Read the model definition and answer for the solid it produces. Units are mm, in the model's axes. Face numbers are marked on the shaded views. A direction names the side the tool comes from. Coordinates: 2 decimals unless noted, no trailing zeros. Loops run counter-clockwise (first coordinate to the right, second up) from the corner with the lowest first, then second, coordinate; pieces in that order, holes last. Notation, with made-up numbers: M 11.25,45.5 L 58.25,45.5 A17 ccw 58.25,69.5 Z; hole C -33.5,62.25 d1. An arc over 180 degrees is marked long. Put each result on its own line as item: value.
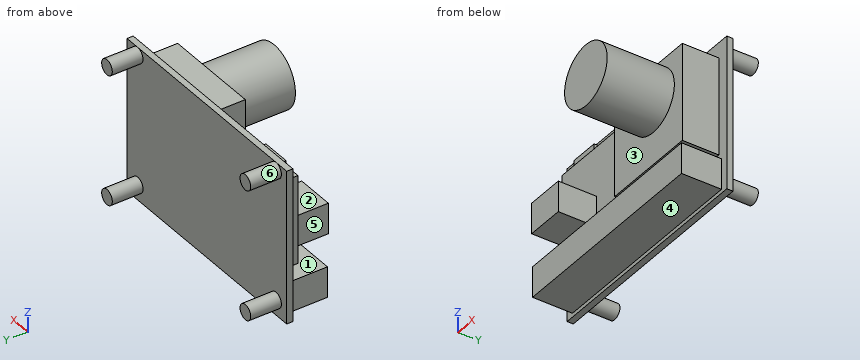
from build123d import *

# Parameters (mm, degrees)
P01_STANDOFF_START             = 28.6
SK_P01_STANDOFF_R              = 2
P01_STANDOFF_DEPTH             = 8
P02_STANDOFF_START             = 28.6
SK_P02_STANDOFF_R              = 2
P02_STANDOFF_DEPTH             = 8
P03_STANDOFF_START             = 28.6
SK_P03_STANDOFF_R              = 2
P03_STANDOFF_DEPTH             = 8
P04_STANDOFF_START             = 28.6
SK_P04_STANDOFF_R              = 2
P04_STANDOFF_DEPTH             = 8
P05_CARRIERBOARD_START         = 27
SK_P05_CARRIERBOARD_W          = 60
SK_P05_CARRIERBOARD_H          = 40
P05_CARRIERBOARD_DEPTH         = 1.6
P06_INA2602COMPUTE_START       = 24.3
SK_P06_INA2602COMPUTE_W        = 22.9
SK_P06_INA2602COMPUTE_H        = 23
P06_INA2602COMPUTE_DEPTH       = 2.7
P07_INA260TERMINALBLOCK_START  = 14.3
SK_P07_INA260TERMINALBLOCK_W   = 10
SK_P07_INA260TERMINALBLOCK_H   = 8
P07_INA260TERMINALBLOCK_DEPTH  = 10
P08_BUCKAD36V50F551V_START     = 17.5
SK_P08_BUCKAD36V50F551V_W      = 25.4
SK_P08_BUCKAD36V50F551V_H      = 25.4
P08_BUCKAD36V50F551V_DEPTH     = 9.5
P09_JSTXHHEADERSFACEDOWN_START = 16.6
SK_P09_JSTXHHEADERSFACEDOWN_W  = 56
SK_P09_JSTXHHEADERSFACEDOWN_H  = 8
P09_JSTXHHEADERSFACEDOWN_DEPTH = 10.4
P10_D2IDEALDIODE_START         = 24.6
SK_P10_D2IDEALDIODE_W          = 7.6
SK_P10_D2IDEALDIODE_H          = 12.7
P10_D2IDEALDIODE_DEPTH         = 2.4
SK_P11_C14700UF25V_R           = 8
P11_C14700UF25V_DEPTH          = 27


with BuildPart() as part:
    # SK_P01_Standoff → P01_Standoff (new body)
    with BuildSketch(Plane(origin=(0, 0, 0), x_dir=(1, 0, 0), z_dir=(0, 1, 0)).offset(P01_STANDOFF_START)):
        with Locations(Location((-26, -18, 0), (0, 0, 270))):
            Circle(SK_P01_STANDOFF_R)
    extrude(amount=P01_STANDOFF_DEPTH)



with BuildPart() as body_2:
    # SK_P02_Standoff → P02_Standoff (new body)
    with BuildSketch(Plane(origin=(0, 0, 0), x_dir=(1, 0, 0), z_dir=(0, 1, 0)).offset(P02_STANDOFF_START)):
        with Locations(Location((-26, 16, 0), (0, 0, 270))):
            Circle(SK_P02_STANDOFF_R)
    extrude(amount=P02_STANDOFF_DEPTH)


with BuildPart() as body_3:
    # SK_P03_Standoff → P03_Standoff (new body)
    with BuildSketch(Plane(origin=(0, 0, 0), x_dir=(1, 0, 0), z_dir=(0, 1, 0)).offset(P03_STANDOFF_START)):
        with Locations(Location((26, -18, 0), (0, 0, 270))):
            Circle(SK_P03_STANDOFF_R)
    extrude(amount=P03_STANDOFF_DEPTH)


with BuildPart() as body_4:
    # SK_P04_Standoff → P04_Standoff (new body)
    with BuildSketch(Plane(origin=(0, 0, 0), x_dir=(1, 0, 0), z_dir=(0, 1, 0)).offset(P04_STANDOFF_START)):
        with Locations(Location((26, 16, 0), (0, 0, 270))):
            Circle(SK_P04_STANDOFF_R)
    extrude(amount=P04_STANDOFF_DEPTH)


with BuildPart() as part_1:
    add(part.part)

    add(body_2.part)  # P05_Carrierboard merges body 2

    add(body_3.part)  # P05_Carrierboard merges body 3

    add(body_4.part)  # P05_Carrierboard merges body 4
    # SK_P05_Carrierboard → P05_Carrierboard (add)
    with BuildSketch(Plane(origin=(0, 0, 0), x_dir=(1, 0, 0), z_dir=(0, 1, 0)).offset(P05_CARRIERBOARD_START)):
        Rectangle(SK_P05_CARRIERBOARD_W, SK_P05_CARRIERBOARD_H)
    extrude(amount=P05_CARRIERBOARD_DEPTH)

    # SK_P06_INA2602compute → P06_INA2602compute (add)
    with BuildSketch(Plane(origin=(0, 0, 0), x_dir=(1, 0, 0), z_dir=(0, 1, 0)).offset(P06_INA2602COMPUTE_START)):
        with Locations((-16.55, -4.5)):
            Rectangle(SK_P06_INA2602COMPUTE_W, SK_P06_INA2602COMPUTE_H)
    extrude(amount=P06_INA2602COMPUTE_DEPTH)

    # SK_P07_INA260terminalblock → P07_INA260terminalblock (add)
    with BuildSketch(Plane(origin=(0, 0, 0), x_dir=(1, 0, 0), z_dir=(0, 1, 0)).offset(P07_INA260TERMINALBLOCK_START)):
        with Locations((-20, 1)):
            Rectangle(SK_P07_INA260TERMINALBLOCK_W, SK_P07_INA260TERMINALBLOCK_H)
    extrude(amount=P07_INA260TERMINALBLOCK_DEPTH)

    # SK_P08_BuckAD36V50F551V → P08_BuckAD36V50F551V (add)
    with BuildSketch(Plane(origin=(0, 0, 0), x_dir=(1, 0, 0), z_dir=(0, 1, 0)).offset(P08_BUCKAD36V50F551V_START)):
        with Locations((14.3, -3.3)):
            Rectangle(SK_P08_BUCKAD36V50F551V_W, SK_P08_BUCKAD36V50F551V_H)
    extrude(amount=P08_BUCKAD36V50F551V_DEPTH)

    # SK_P09_JSTXHheadersfacedown → P09_JSTXHheadersfacedown (add)
    with BuildSketch(Plane(origin=(0, 0, 0), x_dir=(1, 0, 0), z_dir=(0, 1, 0)).offset(P09_JSTXHHEADERSFACEDOWN_START)):
        with Locations((0, 15)):
            Rectangle(SK_P09_JSTXHHEADERSFACEDOWN_W, SK_P09_JSTXHHEADERSFACEDOWN_H)
    extrude(amount=P09_JSTXHHEADERSFACEDOWN_DEPTH)

    # SK_P10_D2idealdiode → P10_D2idealdiode (add)
    with BuildSketch(Plane(origin=(0, 0, 0), x_dir=(1, 0, 0), z_dir=(0, 1, 0)).offset(P10_D2IDEALDIODE_START)):
        with Locations((-20.2, -11.35)):
            Rectangle(SK_P10_D2IDEALDIODE_W, SK_P10_D2IDEALDIODE_H)
    extrude(amount=P10_D2IDEALDIODE_DEPTH)

    # SK_P11_C14700uF25V → P11_C14700uF25V (add)
    with BuildSketch(Plane(origin=(0, 0, 0), x_dir=(1, 0, 0), z_dir=(0, 1, 0))):
        with Locations(Location((16, -7, 0), (0, 0, 270))):
            Circle(SK_P11_C14700UF25V_R)
    extrude(amount=P11_C14700UF25V_DEPTH)


solid = part_1.part
1) Find section A-A, the plane y = 22.5. Write down the section's boundary in (x, z), plus the area to 3 significant figures.
Answer list:
outline: M -28,-19 L 28,-19 L 28,-11 L -28,-11 Z; M -25,-5 L -15,-5 L -15,3 L -25,3 Z; M 1.6,-9.4 L 27,-9.4 L 27,16 L 1.6,16 Z
area: 1,170 mm^2
2) Which of the six approach directions +Z, -Z, +X, -X, +Y, -Y give full straight-line access (tool end or side, diameter ignored) to the marked faces 1, 2 and 3?
Answer list:
face 1: +X, -X, -Y
face 2: +Z, -X, -Y
face 3: -Y
3) Determine the mould class of the marked faces 4, 5 and 6 for opening direction X: released by +X, released by -X, zero draft, split by the parting line, or undercut.
Answer list:
face 4: zero draft
face 5: released by -X
face 6: undercut
4) Find section C-C, the plane z = -16. Write down the section's boundary in (x, y).
Answer list:
outline: M -30,27 L -28,27 L -28,16.6 L 28,16.6 L 28,27 L 30,27 L 30,28.6 L 28,28.6 L 28,36.6 L 24,36.6 L 24,28.6 L -24,28.6 L -24,36.6 L -28,36.6 L -28,28.6 L -30,28.6 Z
5) Find section D-D, the plane x = -6. Write down the section's boundary in (y, z), plus the area to 3 significant figures.
Answer list:
outline: M 16.6,-19 L 27,-19 L 27,-20 L 28.6,-20 L 28.6,20 L 27,20 L 27,16 L 24.3,16 L 24.3,-7 L 27,-7 L 27,-11 L 16.6,-11 Z
area: 209 mm^2
6) Find section B-B, the plane x = 16. Write down the section's boundary in (y, z).
Answer list:
outline: M 0,-1 L 17.5,-1 L 17.5,-9.4 L 27,-9.4 L 27,-11 L 16.6,-11 L 16.6,-19 L 27,-19 L 27,-20 L 28.6,-20 L 28.6,20 L 27,20 L 27,16 L 17.5,16 L 17.5,15 L 0,15 Z
7) Given pin 1 Ø3 at (x, y) = (9, 22.5) entering from +Z; pin 2 Ø10 at (y, z) = (9, 11.5) entering from +X; pin 3 Ø1.2 at (x, y) = (-21.5, 25.5) entering from +Z, each flat-ended and moving along its own axis, determine where each tip first touches the part or whether it passes through.
Answer list:
pin 1: stops at z = 16
pin 2: stops at x = 24
pin 3: stops at z = 17.7
8) Straight lines are drawn through the part: line 1 (Z direction, x = 12, y = 22); line 2 (X direction, y = 25.5, z = -6.5); line 3 (Y direction, x = 20.5, z = 16.5). For each, find the intervals that lie inside material, in ascending order. Write a range as [from, to].
Answer list:
line 1: z = [-19, -11], [-9.4, 16]
line 2: x = [-28, -5.1], [1.6, 27]
line 3: y = [27, 28.6]
